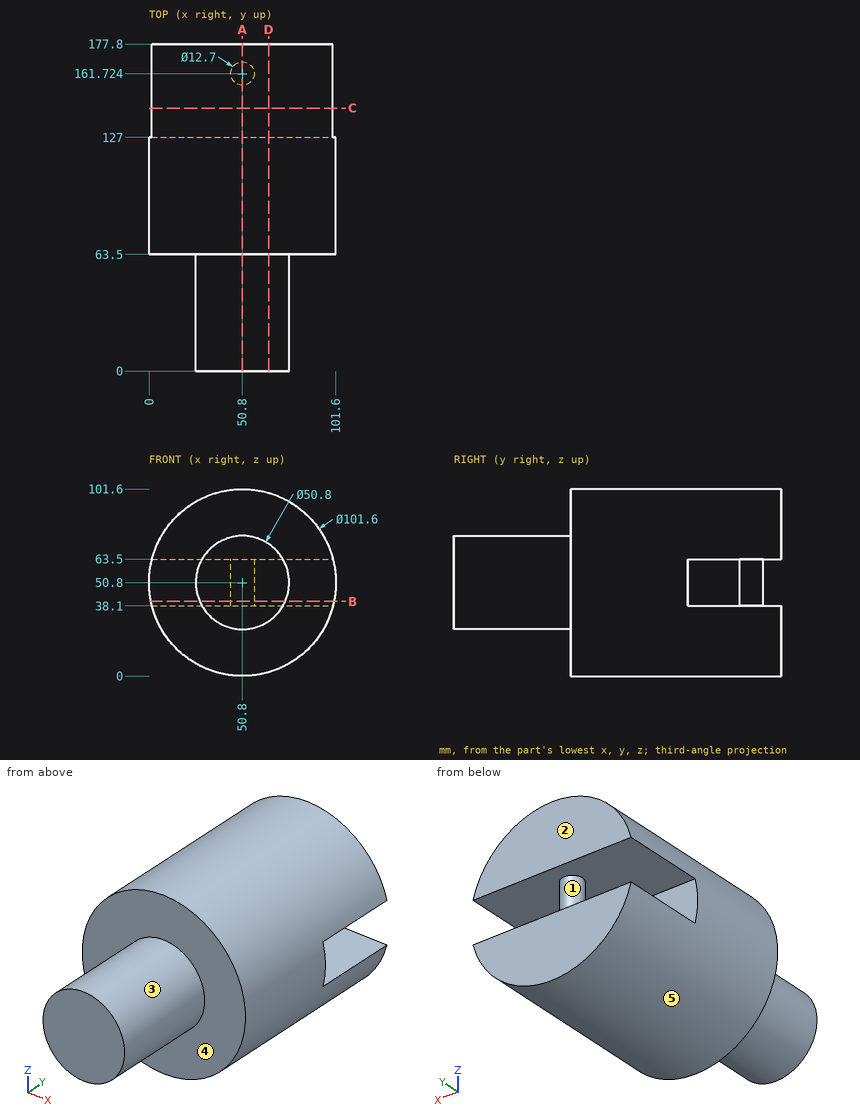
Verification items for this drawing (mm, ordinates from the low corner). A direction names the side the tool comes from. Round coordinates to 2 decimals unless told otherwise and drop trailing zeros. Write each loop counter-clockwise with the first axis right and the second up, starting at its lowest first coordinate (ties: lowest second). Pieces come first, ordered by that corner, then holes. Notation, with made-up numbers: M 52.25,42 L 106.25,42 A15 ccw 106.25,54 Z; hole C 27,77.25 d2. An arc over 180 degrees is marked long. Write item = value, one per line. Start each with the question number.
1. Scan lines: line 1 (Z direction, x = 52, y = 170); line 2 (Z direction, x = 52, y = 30); line 3 (Y direction, x = 62, z = 22.5). Record each from-to range of solid material in increasing order. Write a range as [from, to].
2. Release check for a two-part mould opening along Z. For the marked faces 1, 2 and 3 record: pulls with the +Z half, pulls with the -Z half, needs draft (parallel to the pull), parting line crosses it, or undercut.
3. Section check D-D, the plane x = 65. Record the cut outline in (y, z) (3 decimals).
4. Tool access check on the marked faces 4 and 5. Record the directions out of +Z, -Z, +X, -X, +Y, -Y that give a thin tool (end or side, any length) a straight path to the whole face; none if there is none.
5. Section check C-C, the plane y = 143. Record the cut outline in (x, z), then the cut area to 3 significant figures.
6. Gauge pin test, flat ends, axial feed: pin 1 (4 mm diameter, centred on x = 40, z = 51.5, fed in from +Y); pin 2 (15 mm diameter, centred on x = 35.5, y = 148, fed in from -Z); pin 3 (10 mm diameter, centred on y = 155, z = 80, fed in from -X). Record the tip position at first contact, or that the pin passes through.
7. Section check B-B, the plane z = 40.5. Record the cut outline in (x, y) (3 decimals), then the cut area to 3 significant figures.
8. Section check A-A, the plane x = 50.8. Record the cut outline in (y, z).
Results found:
q1.line_1 = [0.01, 38.1], [63.5, 101.59]
q1.line_2 = [25.43, 76.17]
q1.line_3 = [63.5, 177.8]
q2.face_1 = undercut
q2.face_2 = needs draft
q2.face_3 = parting line crosses it
q3.outline = M 0,29.74 L 63.5,29.74 L 63.5,2.025 L 177.8,2.025 L 177.8,38.1 L 127,38.1 L 127,63.5 L 177.8,63.5 L 177.8,99.575 L 63.5,99.575 L 63.5,71.86 L 0,71.86 Z
q4.face_4 = -Y
q4.face_5 = +Y, -Y
q5.outline = M 1.61,38.1 A50.8 ccw 99.99,38.1 Z; M 1.61,63.5 L 99.99,63.5 A50.8 ccw Z
q5.area = 5,550 mm^2
q6.pin_1 = 127
q6.pin_2 = 0.6
q6.pin_3 = 6.13
q7.outline = M 1.055,63.5 L 27.582,63.5 L 27.582,0 L 74.018,0 L 74.018,63.5 L 100.545,63.5 L 100.545,127 L 1.055,127 Z; C 50.8,161.724 d12.7
q7.area = 9,390 mm^2
q8.outline = M 0,25.4 L 63.5,25.4 L 63.5,0 L 177.8,0 L 177.8,38.1 L 168.07,38.1 L 168.07,63.5 L 177.8,63.5 L 177.8,101.6 L 63.5,101.6 L 63.5,76.2 L 0,76.2 Z; hole M 127,38.1 L 155.37,38.1 L 155.37,63.5 L 127,63.5 Z
